```python
from build123d import *

# Parameters (mm, degrees)
F1_DEPTH      = 25.4
F1_DEPTH_BACK = 25.4
F2_R          = 5.08
F4_D          = 6.35


with BuildPart() as f1:
    # F0 (on Front) → F1 (new body, two sides)
    with BuildSketch(Plane.XZ) as f1_sk:
        Polygon((-76.2, 107.919905), (-101.6, 107.919905), (-101.6, -95.280095), (101.6, -95.280095), (101.6, 107.919905), (76.2, 107.919905), (76.2, -69.880095), (-76.2, -69.880095), align=None)
    extrude(amount=F1_DEPTH)
    extrude(f1_sk.sketch, amount=-F1_DEPTH_BACK)

    # F2
    f2_edges = [f1.edges().sort_by_distance(p)[0] for p in [
        (-88.9, -25.4, 107.919905),
        (-88.9, 25.4, 107.919905),
        (88.9, -25.4, 107.919905),
        (88.9, 25.4, 107.919905),
        (-76.2, 0, -69.880095),
        (76.2, 0, -69.880095),
    ]]
    fillet(f2_edges, radius=F2_R)

    # F4 (through all)
    with Locations(Plane(origin=(-101.6, 0, 0), x_dir=(0, -1, 0), z_dir=(-1, 0, 0))):
        with Locations((0, 82.519905)):
            Hole(F4_D / 2)


solid = f1.part
```
Can you work these out from the model? Positions are in its coordinate system, mm. A direction names the side the tool comes from. Give positions to 0.01 mm unless a question says otherwise; leave off trailing zeros. Order: outer loops, then holes, each group sorted by start corner. A loop starts at its lowest first (then second) coordinate and runs counter-clockwise, first axis right, second up. Notation, with made-up numbers: M 87.5,71 L 92.5,71 A22 cw 92.5,85 Z; hole C 65,-37 d7. An arc over 180 degrees is marked long. One line per item, written item: value.
1) On a 3-axis mill with a long thin cutter (end or side, diameter ignored), from which of +Z, -Z, +X, -X, +Y, -Y can I reach the whole of each face in a straight line? I mean faces 5 (the face through (0, -25.4, -76)), 6 (the face through (74.672, 0.356, -68.431)). Say none if no direction works.
Answer sheet:
face 5: +Z, -Z, +X, -X, -Y
face 6: +Z, +Y, -Y
2) Please list where these lines run through material, in increasing order: line 1 along X through (y, z) = (23.5, 48.5); line 2 along Z through (x, y) = (-85.5, 0); line 3 along Z through (x, y) = (5, 9).
Answer sheet:
line 1: x = -101.6 to -76.2, 76.2 to 101.6
line 2: z = -95.28 to 79.34, 85.69 to 107.92
line 3: z = -95.28 to -69.88
3) For P1, Ø8, axis at x = 53.5, y = 1.5, coming from the +Z side, with a flat end and sliding along its axis, tell me the tip position at first contact or that it passes through.
Answer sheet:
P1: stops at z = -69.88
4) I want a section at C-C, the plane y = -17. List the corners of the cut face in (x, z) for me, plus the area to 3 significant figures.
Answer sheet:
outline: M -101.6,-95.28 L 101.6,-95.28 L 101.6,107.92 L 76.2,107.92 L 76.2,-64.8 A5.08 cw 71.12,-69.88 L -71.12,-69.88 A5.08 cw -76.2,-64.8 L -76.2,107.92 L -101.6,107.92 Z
area: 14,200 mm^2
5) I want a section at A-A, the plane z = 69.5. List the corners of the cut face in (x, y) for me.
Answer sheet:
outline: M -101.6,-25.4 L -76.2,-25.4 L -76.2,25.4 L -101.6,25.4 Z; M 76.2,-25.4 L 101.6,-25.4 L 101.6,25.4 L 76.2,25.4 Z
6) I want a section at B-B, the plane y = 0. List the corners of the cut face in (x, z) for me, plus the area to 3 significant figures.
Answer sheet:
outline: M -101.6,-95.28 L 101.6,-95.28 L 101.6,79.34 L 76.2,79.34 L 76.2,-64.8 A5.08 cw 71.12,-69.88 L -71.12,-69.88 A5.08 cw -76.2,-64.8 L -76.2,79.34 L -101.6,79.34 Z; M -101.6,85.69 L -76.2,85.69 L -76.2,107.92 L -101.6,107.92 Z; M 76.2,85.69 L 101.6,85.69 L 101.6,107.92 L 76.2,107.92 Z
area: 13,900 mm^2
7) I want a section at D-D, the plane x = -14.5. List the corners of the cut face in (y, z) for me.
Answer sheet:
outline: M -25.4,-95.28 L 25.4,-95.28 L 25.4,-69.88 L -25.4,-69.88 Z
8) We'd pull the mould along X, two halves only. Please class faces 1 (the face through (88.722, 23.872, 106.471)), 2 (the face through (-74.751, 0.356, -68.352)), 3 (the face through (-101.6, 0, 8)), 4 (the face through (76.2, 0, 23)): released by +X, released by -X, zero draft, split by the parting line, or undercut.
Answer sheet:
face 1: zero draft
face 2: undercut
face 3: released by -X
face 4: undercut
